Autodesk Inventor part; units mm, degrees
ref_plane "YZ Plane" through (0, 0, 0) normal (1, 0, 0) x (0, 1, 0)
ref_plane "XZ Plane" through (0, 0, 0) normal (0, 1, 0) x (-1, 0, 0)
ref_plane "XY Plane" through (0, 0, 0) normal (0, 0, 1) x (1, 0, 0)
sketch "Sketch1" plane through (0, 0, 0) normal (0, 1, 0) x (-1, 0, 0)
  line L0 (10.5834, 13.2197) -> (-47.9966, 13.2197)
  line L1 (-47.9966, 13.2197) -> (-47.9966, -11.7803)
  line L2 (-47.9966, -11.7803) -> (10.5834, -11.7803)
  line L3 (10.5834, -11.7803) -> (10.5834, 13.2197)
  circle A0 centre (5.5834, -7.8803) radius 1.55
  circle A1 centre (5.5834, 2.1197) radius 1.55
  circle A2 centre (-4.4166, 2.1197) radius 1.55
  circle A3 centre (-37.9966, 8.2197) radius 1.55
  circle A4 centre (-37.9966, -6.7803) radius 1.55
  point P0 (0, 0)
  dimension "d0" = 3.1
  dimension "d1" = 3.9
  dimension "d4" = 10
  dimension "d11" = 10
  dimension "d16" = 25
  dimension "d17" = 5
  dimension "d18" = 58.58
  dimension "d19" = 3.1
  dimension "d20" = 10
  dimension "d23" = 15
  dimension "d28" = 5
extrude "Extrusion1" add sketch "Sketch1" along normal mid plane 4
sketch "Sketch2" plane through (47.9966, 2, -11.7803) normal (0, 0, -1) x (-1, 0, 0)
  arc A0 (40.37, 0) -> (40.62, 0) centre (40.495, 0) ccw
  line L0 (0, 0) -> (58.58, 0)
  line L1 (58.58, -4) -> (58.58, 0)
  circle A1 centre (20, 0) radius 0.125
  line L2 (0, -4) -> (0, 0)
  point P0 (47.9966, -2)
  point P1 (58.58, -2)
  point P2 (20.125, 0)
  point P3 (19.875, 0)
  dimension "d31" = 0.25
  dimension "d34" = 18.085
  dimension "d35" = 0.25
  dimension "d36" = 20
extrude "Extrusion2" cut sketch "Sketch2" against normal up to surface (25 mm away) contours L0 A0 | A1 L0 picked at (20, -0.0736)
fillet "Fillet1" radius 0.1 4 edges at (7.6266, 2, 0.7197) (7.3766, 2, 0.7197) (28.1216, 2, 0.7197) (27.8716, 2, 0.7197)
fillet "Fillet2" radius 5 1 edges at (-10.5834, 0, 13.2197)
properties part number "GVS_Plate"
The listing builds one solid part. Answer for the finished solid, in the listing's coordinates (mm). Round coordinates to 2 decimals unless told otherwise and drop trailing zeros. Order: outer loops, then holes, each group sorted by start corner. A loop starts at its lowest first (then second) coordinate and runs counter-clockwise, first axis right, second up. Notation, with made-up numbers: (4.5, 66.5) -> (62.5, 66.5) arc R6 ccw to (62.5, 77.5) -> close; hole circle Ø5 at (-39, -21). An arc over 180 degrees is marked (long way). Answer as CSV lines item,"result".
Q1. A cutting plane is placed at B-B on y = -1.3. Determine the outline of the cut face in (x, z), plus the area to 3 significant figures.
Computed values:
outline,"(-10.58, -11.78) -> (48, -11.78) -> (48, 13.22) -> (-5.58, 13.22) arc R5 ccw to (-10.58, 8.22) -> close; hole circle Ø3.1 at (-5.58, -7.88); hole circle Ø3.1 at (-5.58, 2.12); hole circle Ø3.1 at (4.42, 2.12); hole circle Ø3.1 at (38, -6.78); hole circle Ø3.1 at (38, 8.22)"
area,"1,420 mm^2"
Q2. A cutting plane is placed at C-C on z = -5.75. Determine the outline of the cut face in (x, y) (3 decimals), plus the area to 3 significant figures.
Computed values:
outline,"(-10.583, -2) -> (36.839, -2) -> (36.839, 2) -> (28.198, 2) arc R0.1 ccw to (28.109, 1.944) arc R0.125 cw to (27.885, 1.944) arc R0.1 ccw to (27.795, 2) -> (7.703, 2) arc R0.1 ccw to (7.614, 1.944) arc R0.125 cw to (7.39, 1.944) arc R0.1 ccw to (7.3, 2) -> (-10.583, 2) -> close; (39.155, -2) -> (47.997, -2) -> (47.997, 2) -> (39.155, 2) -> close"
area,"225 mm^2"
Q3. A cutting plane is placed at A-A on z = 7.25. Determine the outline of the cut face in (x, y) (3 decimals).
Computed values:
outline,"(-10.583, -2) -> (36.787, -2) -> (36.787, 2) -> (28.198, 2) arc R0.1 ccw to (28.109, 1.944) arc R0.125 cw to (27.885, 1.944) arc R0.1 ccw to (27.795, 2) -> (7.703, 2) arc R0.1 ccw to (7.614, 1.944) arc R0.125 cw to (7.39, 1.944) arc R0.1 ccw to (7.3, 2) -> (-10.583, 2) -> close; (39.206, -2) -> (47.997, -2) -> (47.997, 2) -> (39.206, 2) -> close"
Q4. Consider line 1 (X direction, y = -1.8, z = 1.75); line 2 (Z direction, x = -5, y = -0.95); line 3 (X direction, y = 1.2, z = 7.5). Determine where each line is inside the solid, lowest interval first. Write a range as from..to.
Computed values:
line 1,"x = -10.58..-7.09, -4.08..2.91, 5.92..48"
line 2,"z = -11.78..-9.32, -6.44..0.68, 3.56..13.22"
line 3,"x = -10.58..36.62, 39.37..48"
Q5. For a pull along Z with two mould halves and no side action, classify faces 1 (the flat face through (-2, 2, 1)), 2 (the cylindrical face through (-9.158, 0.028, 11.716)), 3 (the cylindrical face through (2.94, -0.03, 1.65)), 4 (the flat face through (19, 0, -11.78)) as +Z half, -Z half, draft (parallel to the pull), parting line (faces both ways), or undercut.
Computed values:
face 1,"draft"
face 2,"+Z half"
face 3,"undercut"
face 4,"-Z half"
Q6. Given pin 1 (1.9 mm diameter, centred on x = 38, z = 8.22, fed in from -Y), flat-ended and moving along its own axis, determine where the tip first touches the part or whether it passes through.
Computed values:
pin 1,"passes through"
